from build123d import *

# Parameters (mm, degrees)
SKETCH1_W           = 20
SKETCH1_H           = 20
BOSS_EXTRUDE1_DEPTH = 5
SKETCH2_R           = 4.05
CUT_EXTRUDE1_DEPTH  = 18.320508076
SKETCH3_R           = 2
CUT_EXTRUDE2_DEPTH  = 23.912878475
SKETCH4_R           = 0.5
CUT_EXTRUDE3_DEPTH  = 10
CHAMFER1_SIZE       = 0.5


with BuildPart() as part:
    # Sketch1 → Boss-Extrude1 (new, symmetric)
    with BuildSketch(Plane(origin=(0, 0, 0), x_dir=(1, 0, 0), z_dir=(0, 1, 0))):
        Rectangle(SKETCH1_W, SKETCH1_H)
    extrude(amount=BOSS_EXTRUDE1_DEPTH, both=True)

    # Sketch2 → Cut-Extrude1 (cut, through all)
    with BuildSketch(Plane(origin=(0, 5, 0), x_dir=(1, 0, 0), z_dir=(0, 1, 0))):
        with Locations(Location((0, -3, 0), (0, 0, 270))):
            Circle(SKETCH2_R)
    extrude(amount=-CUT_EXTRUDE1_DEPTH, mode=Mode.SUBTRACT)

    # Sketch3 → Cut-Extrude2 (cut, through all)
    with BuildSketch(Plane(origin=(10, 0, 0), x_dir=(0, 0, -1), z_dir=(1, 0, 0))):
        with Locations((6.442090049, 0)):
            Circle(SKETCH3_R)
    extrude(amount=-CUT_EXTRUDE2_DEPTH, mode=Mode.SUBTRACT)

    # Sketch4 → Cut-Extrude3 (cut)
    with BuildSketch(Plane(origin=(10, 0, 0), x_dir=(0, 0, -1), z_dir=(1, 0, 0))):
        with Locations((2.442090049, 0)):
            Circle(SKETCH4_R)
    extrude(amount=-CUT_EXTRUDE3_DEPTH, mode=Mode.SUBTRACT)

    # Chamfer1
    chamfer1_edges = [part.edges().sort_by_distance(p)[0] for p in [
        (-10, 5, 0),
        (0, 5, 10),
        (10, 5, 0),
        (0, -5, 10),
        (-10, -5, 0),
        (0, -5, -10),
        (10, -5, 0),
        (10, 0, 10),
        (-10, 0, 10),
        (-10, 0, -10),
        (10, 0, -10),
        (0, 5, -10),
    ]]
    chamfer(chamfer1_edges, length=CHAMFER1_SIZE)


solid = part.part
Read the model definition and answer for the solid it produces. Units are mm, in the model's axes. A direction names the side the tool comes from. Give positions to 0.01 mm unless a question says otherwise; leave off trailing zeros. Loops run counter-clockwise (first coordinate to the right, second up) from the corner with the lowest first, then second, coordinate; pieces in that order, holes last. Notation, with made-up numbers: (41, 53.25) -> (89, 53.25) arc R26 ccw to (89, 80.25) -> close; hole circle Ø6 at (2.25, 69.25). An arc over 180 degrees is marked (long way). Use a Markdown table: item, result.
Q1. Determine the mould class of faces 1 (the face through (10, 0, 0)), 2 (the face through (0, 0, -10)), 3 (the face through (0, 0, -2.4)), 4 (the face through (-3.593, 0.07, 4.869)) for opening direction Z: pulls with the +Z half, pulls with the -Z half, needs draft (parallel to the pull), parting line crosses it, or undercut.
Solved:
| item | result |
|---|---|
| face 1 | needs draft |
| face 2 | pulls with the -Z half |
| face 3 | undercut |
| face 4 | undercut |
Q2. Section B-B, the plane z = 3 is taken. Determine the outline of the cut face in (x, y), then the cut area to 4 significant figures.
Solved:
| item | result |
|---|---|
| outline | (-10, -4.5) -> (-9.5, -5) -> (-4.05, -5) -> (-4.05, 5) -> (-9.5, 5) -> (-10, 4.5) -> close; (4.05, -5) -> (9.5, -5) -> (10, -4.5) -> (10, 4.5) -> (9.5, 5) -> (4.05, 5) -> close |
| area | 118.5 mm^2 |
Q3. Section A-A, the plane y = 0 is taken. Determine the outline of the cut face in (x, z).
Solved:
| item | result |
|---|---|
| outline | (-10, -9.5) -> (-9.5, -10) -> (9.5, -10) -> (10, -9.5) -> (10, -8.44) -> (-10, -8.44) -> close; (-10, -4.44) -> (10, -4.44) -> (10, -2.94) -> (0, -2.94) -> (0, -1.94) -> (10, -1.94) -> (10, 9.5) -> (9.5, 10) -> (-9.5, 10) -> (-10, 9.5) -> close; hole circle Ø8.1 at (0, 3) |
Q4. Section C-C, the plane x = 6 is taken. Determine the outline of the cut face in (y, z), then the cut area to 3 significant figures.
Solved:
| item | result |
|---|---|
| outline | (-5, -9.5) -> (-4.5, -10) -> (4.5, -10) -> (5, -9.5) -> (5, 9.5) -> (4.5, 10) -> (-4.5, 10) -> (-5, 9.5) -> close; hole circle Ø4 at (0, -6.44); hole circle Ø1 at (0, -2.44) |
| area | 186 mm^2 |
Q5. Section D-D, the plane y = 3.5 is taken. Determine the outline of the cut face in (x, z), then the cut area to 3 significant figures.
Solved:
| item | result |
|---|---|
| outline | (-10, -9.5) -> (-9.5, -10) -> (9.5, -10) -> (10, -9.5) -> (10, 9.5) -> (9.5, 10) -> (-9.5, 10) -> (-10, 9.5) -> close; hole circle Ø8.1 at (0, 3) |
| area | 348 mm^2 |
Q6. A tool of negligible diameter and unlimited length cuts with its end or side. For faces 5 (the face through (5.07, 0.022, -1.943)), 6 (the face through (0.14, -1.952, -6.009)), from which of +Z, -Z, +X, -X, +Y, -Y can it reach the whole face along a straight path? Write none if from no direction.
Solved:
| item | result |
|---|---|
| face 5 | +X |
| face 6 | +X, -X |
Q7. Find the intervals of material crossed by line 1 along X through (y, z) = (2.25, 3); line 2 along Z through (x, y) = (2, -0.75); line 3 along Z through (x, y) = (2.25, -1), in increasing order.
Solved:
| item | result |
|---|---|
| line 1 | x = -10 to -4.05, 4.05 to 10 |
| line 2 | z = -10 to -8.3, -4.59 to -0.52, 6.52 to 10 |
| line 3 | z = -10 to -8.17, -4.71 to -0.37, 6.37 to 10 |
